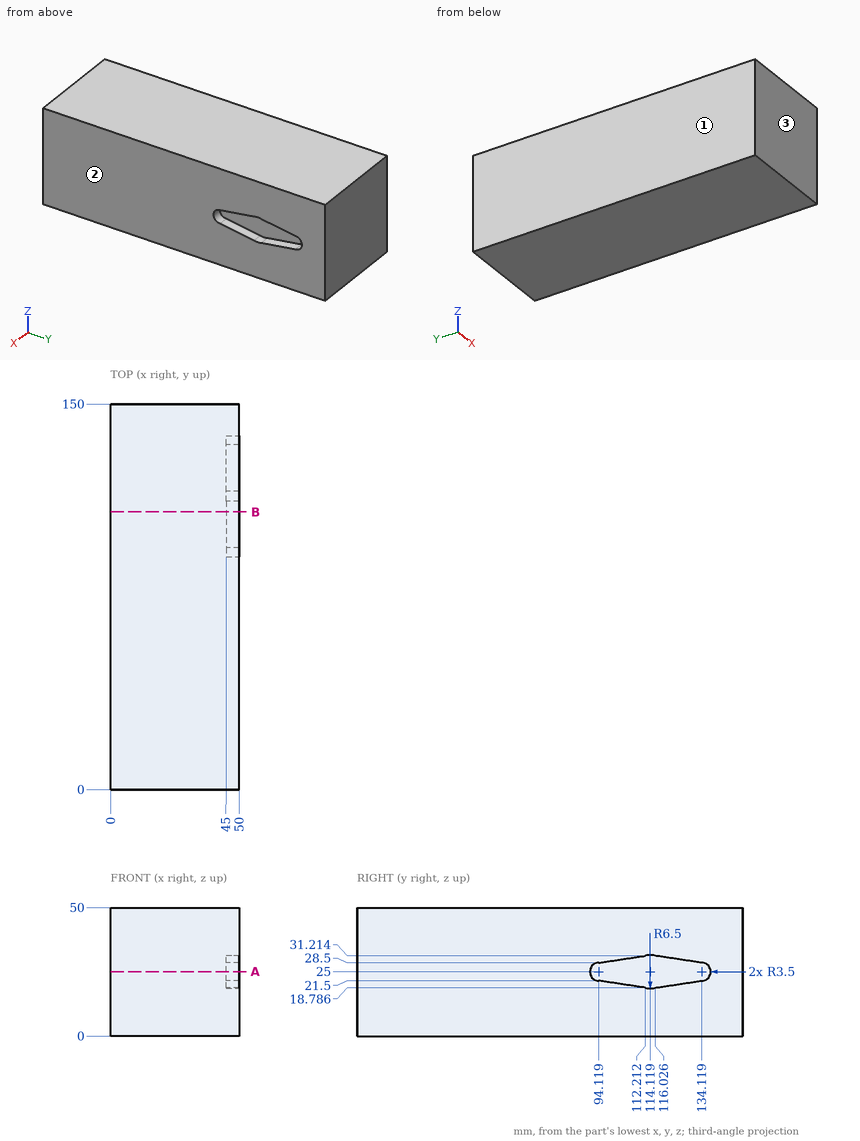
Source: three-view drawing plus pictorial views. Frame: mm from the lowest corner of the part. Give positions to 0.01 mm unless a question says otherwise; leave off trailing zeros. Loops run counter-clockwise (first coordinate to the right, second up) from the corner with the lowest first, then second, coordinate; pieces in that order, holes last.
1) Section query B-B on y = 108. Return the cut outline in (x, z).
A:
outline: (0, 0) - (50, 0) - (50, 19.42) - (45, 19.42) - (45, 30.58) - (50, 30.58) - (50, 50) - (0, 50) - close
2) Line query: L1, parallel to Y at x = 47.5, z = 24 (3 decimals). Output: solid intervals per line, ascending.
A:
L1: y = 0 to 90.765, 137.473 to 150
3) Section query A-A on z = 25. Return the cut outline in (x, y), and give its area (4 significant figures).
A:
outline: (0, 0) - (50, 0) - (50, 90.62) - (45, 90.62) - (45, 137.62) - (50, 137.62) - (50, 150) - (0, 150) - close
area: 7,265 mm2
4) Mould query, pull axis X, two halves, no side actions, for the marked faces 1, 2 and 3. Classes: released by +X, released by -X, zero draft, split by the parting line, or undercut.
A:
face 1: released by -X
face 2: released by +X
face 3: zero draft
5) Contact query for a flat-ended pin moving along its axis: pin 1 (10.5 mm diameter, centred on y = 117.5, z = 25.5, fed in from +X). Output: stop coordinate, or through.
A:
pin 1: stops at x = 45
